Work out the finished part from the listing and answer in its coordinate system (mm). Face numbers are marked on the shaded views. A direction names the side the tool comes from. Coordinates: 2 decimals unless noted, no trailing zeros. Order: outer loops, then holes, each group sorted by start corner. A loop starts at its lowest first (then second) coordinate and runs counter-clockwise, first axis right, second up. Notation, with made-up numbers: M 48,-3 L 52,-3 A20 ccw 52,13 Z; hole C 4.25,84.25 d11. An arc over 180 degrees is marked long. Use a Markdown table: item, result.
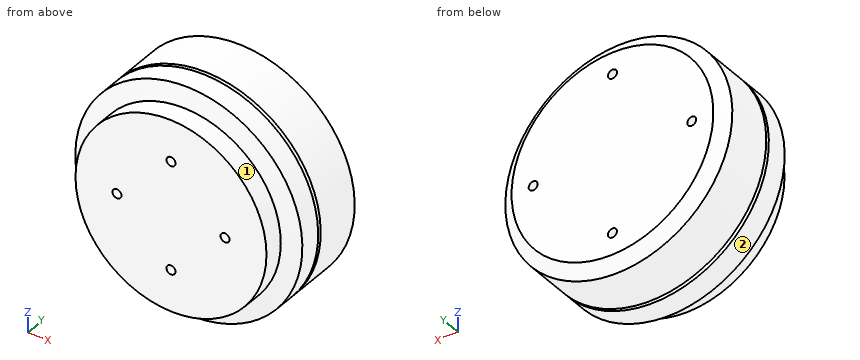
from build123d import *

# Parameters (mm, degrees)
M3X0_5_TAPPED_HOLE1_D     = 2.5
M3X0_5_TAPPED_HOLE1_DEPTH = 6
M3X0_5_TAPPED_HOLE1_TIP   = 0.751075774
M3X0_5_TAPPED_HOLE2_D     = 2.5
M3X0_5_TAPPED_HOLE2_DEPTH = 8.5
M3X0_5_TAPPED_HOLE2_TIP   = 0.751075774


with BuildPart() as part:
    # Sketch1 → Revolve1 (revolve)
    with BuildSketch(Plane.XY, mode=Mode.PRIVATE) as revolve1_sk:
        Polygon((0, 0), (0, 30), (-28, 30), (-31.5, 27.5), (-31.5, 14.2), (-29.5, 14.2), (-29.5, 13.2), (-31.5, 13.2), (-31.5, 7), (-26.5, 5.6), (-26.5, 0), align=None)
    revolve(revolve1_sk.sketch.rotate(Axis((0, 0, 0), (0, -1, 0)), 270), axis=Axis((0, 0, 0), (0, -1, 0)))

    # M3x0.5 Tapped Hole1
    with Locations(Plane(origin=(0, 30, 0), x_dir=(1, 0, 0), z_dir=(0, 1, 0))):
        with Locations((0, 22), (0, -22), (22, 0), (-22, 0)):
            Hole(M3X0_5_TAPPED_HOLE1_D / 2, depth=M3X0_5_TAPPED_HOLE1_DEPTH)
            with Locations((0, 0, -(M3X0_5_TAPPED_HOLE1_DEPTH + M3X0_5_TAPPED_HOLE1_TIP / 2))):  # 118° drill point
                Cone(0, M3X0_5_TAPPED_HOLE1_D / 2, M3X0_5_TAPPED_HOLE1_TIP, mode=Mode.SUBTRACT)

    # M3x0.5 Tapped Hole2
    with Locations(Plane(origin=(0, 0, 0), x_dir=(-1, 0, 0), z_dir=(0, -1, 0))):
        with Locations((0, 15), (0, -15), (15, 0), (-15, 0)):
            Hole(M3X0_5_TAPPED_HOLE2_D / 2, depth=M3X0_5_TAPPED_HOLE2_DEPTH)
            with Locations((0, 0, -(M3X0_5_TAPPED_HOLE2_DEPTH + M3X0_5_TAPPED_HOLE2_TIP / 2))):  # 118° drill point
                Cone(0, M3X0_5_TAPPED_HOLE2_D / 2, M3X0_5_TAPPED_HOLE2_TIP, mode=Mode.SUBTRACT)


solid = part.part
(1) A cutting plane is placed at B-B (y = 21.25). Determine the outline of the cut face in (x, z), then the cut area to 3 significant figures.
Conclusion:
| item | result |
|---|---|
| outline | C 0,0 d63 |
| area | 3,120 mm2 |
(2) A cutting plane is placed at A-A (y = 26). Determine the outline of the cut face in (x, z).
Conclusion:
| item | result |
|---|---|
| outline | C 0,0 d63; hole C -22,0 d2.5; hole C 0,-22 d2.5; hole C 0,22 d2.5; hole C 22,0 d2.5 |
(3) Straight lines are drawn through the part: L1, parallel to Z at x = -1, y = 4.25; L2, parallel to Z at x = 15, y = 4; L3, parallel to Z at x = 17, y = 27. For each, find the intervals that lie inside material, in ascending order.
Conclusion:
| item | result |
|---|---|
| L1 | -26.48 to -15.75, -14.25 to 14.25, 15.75 to 26.48 |
| L2 | -21.85 to -1.25, 1.25 to 21.85 |
| L3 | -26.52 to 26.52 |
(4) Given P1, Ø2, axis at x = -21, y = 18.5, coming from the +Z side; P2, Ø12, axis at y = 13.5, z = 3.5, coming from the -X side; P3, Ø12, axis at x = 23, y = 17.5, coming from the -Z side, each flat-ended and moving along its own axis, determine where each tip first touches the part or whether it passes through.
Conclusion:
| item | result |
|---|---|
| P1 | z = 24.34 |
| P2 | x = -31.5 |
| P3 | z = -26.52 |
(5) Which of the six approach directions +Z, -Z, +X, -X, +Y, -Y give full straight-line access (tool end or side, diameter ignored) to the marked faces 1 and 2?
Conclusion:
| item | result |
|---|---|
| face 1 | -Y |
| face 2 | +Y, -Y |
